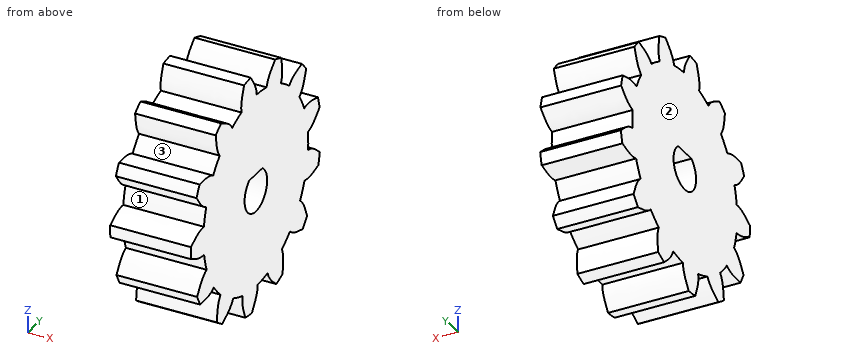
from build123d import *

# Parameters (mm, degrees)
SKETCH3_R           = 12.090863095
BOSS_EXTRUDE1_DEPTH = 10
BOSS_EXTRUDE2_DEPTH = 10
CIRPATTERN1_COUNT   = 13
CUT_EXTRUDE1_DEPTH  = 24.435008607


with BuildPart() as part:
    # Sketch3 → Boss-Extrude1 (new body)
    with BuildSketch(Plane.YZ):
        with Locations(Location((0, 0, 0), (0, 0, 270))):
            Circle(SKETCH3_R)
    extrude(amount=BOSS_EXTRUDE1_DEPTH)

    # Sketch4 → Boss-Extrude2 (add)
    with BuildSketch(Plane.YZ):
        with BuildLine():
            ThreePointArc((-1.195976025, 14.952245361), (-1.957892883, 14.871672921), (-2.714701737, 14.752301328))
            add(Edge.make_bspline(
                [(-2.714701737, 14.752301328), (-3.072545731, 13.791794486), (-3.565367762, 12.687541268), (-3.309213228, 11.62919078)],
                knots=[0.053106957, 0.053106957, 0.053106957, 0.053106957, 1.037972429, 1.037972429, 1.037972429, 1.037972429], degree=3))
            ThreePointArc((-3.309213228, 11.62919078), (-1.57817432, 11.987424085), (0.186598469, 12.089423121))
            add(Edge.make_bspline(
                [(-1.195976025, 14.952245361), (-0.601727805, 14.117083837), (0.160103486, 13.178008863), (0.186598469, 12.089423121)],
                knots=[0.053106957, 0.053106957, 0.053106957, 0.053106957, 1.037972429, 1.037972429, 1.037972429, 1.037972429], degree=3))
        make_face()
    boss_extrude2 = extrude(amount=BOSS_EXTRUDE2_DEPTH)

    # CirPattern1: Boss-Extrude2 ×13 about axis
    cirpattern1_axis = Axis((10, 0, 0), (1, 0, 0))
    for i in range(1, CIRPATTERN1_COUNT):
        add(boss_extrude2.rotate(cirpattern1_axis, i * 360 / CIRPATTERN1_COUNT))

    # Sketch5 → Cut-Extrude1 (cut, through all)
    with BuildSketch(Plane.YZ.offset(10)):
        with BuildLine():
            Line((-1.532970972, 2.1), (1.532970972, 2.1))
            ThreePointArc((1.532970972, 2.1), (0, -2.6), (-1.532970972, 2.1))
        make_face()
    extrude(amount=-CUT_EXTRUDE1_DEPTH, mode=Mode.SUBTRACT)


solid = part.part
Part model, mm, in its own coordinate system. Face numbers are marked on the shaded views. Give positions to 0.01 mm unless a question says otherwise; leave off trailing zeros. Order: outer loops, then holes, each group sorted by start corner. A loop starts at its lowest first (then second) coordinate and runs counter-clockwise, first axis right, second up. Notation, with made-up numbers: (-31.5, 72.25) - (-19.5, 72.25) arc R29 ccw to (-19.5, 105.25) - close; hole circle Ø7 at (51, 25.5). An arc over 180 degrees is marked (long way). Use a Markdown table: item, result.
1) Saw through at A-A on z = 0. List the corners of the cut face in (x, y), plus the area to 3 significant figures.
Checked values:
| item | result |
|---|---|
| outline | (0, -15) - (10, -15) - (10, -2.6) - (0, -2.6) - close; (0, 2.6) - (10, 2.6) - (10, 12.09) - (0, 12.09) - close |
| area | 219 mm² |
2) Saw through at B-B on y = 5.25. List the corners of the cut face in (x, z), plus the area to 3 significant figures.
Checked values:
| item | result |
|---|---|
| outline | (0, -14.05) - (10, -14.05) - (10, 14.05) - (0, 14.05) - close |
| area | 281 mm² |
3) Two-plate mould, pull along Z, no slides. Class the marked faces 1, 2 and 3: +Z half, -Z half, draft (parallel to the pull), parting line (faces both ways), or undercut.
Checked values:
| item | result |
|---|---|
| face 1 | undercut |
| face 2 | draft |
| face 3 | undercut |
4) Probe L1, parallel to Y at x = 6.75, z = 0; L2, parallel to Z at x = 8.25, y = 10.5; L3, parallel to Y at x = 6, z = -1. List the from-to ranges inside material, lowest first. Write a range as from..to.
Checked values:
| item | result |
|---|---|
| L1 | -15..-2.6, 2.6..12.09 |
| L2 | -10.33..-6.77, -5.99..5.99, 7.13..10.59 |
| L3 | -14.81..-2.4, 2.4..12.05 |
5) Flat gauge pins, fed straight in: P1, Ø2.5, axis at x = 3, y = 0.5, coming from the -Z side; P2, Ø3, axis at x = 5.5, z = 1, coming from the +Y side; P3, Ø1, axis at x = 4.5, z = -9.5, coming from the +Y side; P4, Ø4, axis at y = 0, z = 0, coming from the +X side. Where does each tip first touch, or does it go through?
Checked values:
| item | result |
|---|---|
| P1 | z = -14.76 |
| P2 | y = 14.17 |
| P3 | y = 11.81 |
| P4 | through |
